Source: CAD feature listing. Evaluate the final solid. Frame: model axes, mm. Face numbers are marked on the shaded views. A direction names the side the tool comes from. Round coordinates to 2 decimals unless told otherwise and drop trailing zeros. Write each loop counter-clockwise with the first axis right and the second up, starting at its lowest first coordinate (ties: lowest second). Pieces come first, ordered by that corner, then holes. Notation, with made-up numbers: M 70,-31.5 L 83,-31.5 A21 ccw 83,-3.5 Z; hole C 21,-18.75 d5. An arc over 180 degrees is marked long. Answer in a Markdown table with one row per item.
from build123d import *

# Parameters (mm, degrees)
F0_W     = 30
F0_H     = 70
F1_DEPTH = 24
F2_W     = 60
F2_H     = 8.4
F3_DEPTH = 30.001
F5_DEPTH = 20
F6_W     = 20
F6_H     = 5
F7_DEPTH = 8
F9_DEPTH = 75
F10_R    = 5
F11_R    = 2.5
F12_R    = 2.5


with BuildPart() as f1:
    # F0 (on Top) → F1 (new body)
    with BuildSketch(Plane.XY):
        with Locations((15, -35)):
            Rectangle(F0_W, F0_H)
    extrude(amount=F1_DEPTH)

    # F2 (on face) → F3 (cut, through all)
    with BuildSketch(Plane(origin=(0, 0, 0), x_dir=(0, -1, 0), z_dir=(-1, 0, 0))):
        with Locations((40, 12.1)):
            Rectangle(F2_W, F2_H)
    extrude(amount=-F3_DEPTH, mode=Mode.SUBTRACT)

    # F4 (on Right) → F5 (join)
    with BuildSketch(Plane.YZ):
        Polygon((0, -145), (0, 0), (-12, 0), (-12, -92.6724137931), (-12, -125), (-12, -145), align=None)
        Polygon((-12, -125), (-12, -92.6724137931), (-55, 0), (-70, 0), align=None)
    extrude(amount=F5_DEPTH)

    # F6 (on face) → F7 (join)
    with BuildSketch(Plane(origin=(0, 0, 0), x_dir=(-1, 0, 0), z_dir=(0, 1, 0))):
        with Locations((-10, -142.5)):
            Rectangle(F6_W, F6_H)
    extrude(amount=F7_DEPTH)

    # F8 (on face) → F9 (cut)
    with BuildSketch(Plane.XY.offset(-140)):
        with BuildLine():
            ThreePointArc((0, -3.8196601125), (4.647668654, -0.9874146153), (10.0000000012, 0))
            Line((10.0000000012, 0), (0, 0))
            Line((0, 0), (0, -3.8196601125))
        make_face()
        with BuildLine():
            ThreePointArc((10.0000000012, 0), (15.6425875311, -1.1017552924), (20.4562749714, -4.2451725387))
            Line((20.4562749714, -4.2451725387), (20.4562749714, 0))
            Line((20.4562749714, 0), (20, 0))
            Line((20, 0), (10.0000000012, 0))
        make_face()
    extrude(amount=F9_DEPTH, mode=Mode.SUBTRACT)

    # F10
    f10_edges = [f1.edges().sort_by_distance(p)[0] for p in [
        (0, 8, -142.5),
        (20, 8, -142.5),
    ]]
    fillet(f10_edges, radius=F10_R)

    # F11
    f11_edges = [f1.edges().sort_by_distance(p)[0] for p in [
        (0, 0, -20.5),
        (20, 0, -32.5),
    ]]
    fillet(f11_edges, radius=F11_R)

    # F12
    f12_edges = [f1.edges().sort_by_distance(p)[0] for p in [
        (30, 0, 12),
    ]]
    fillet(f12_edges, radius=F12_R)


solid = f1.part
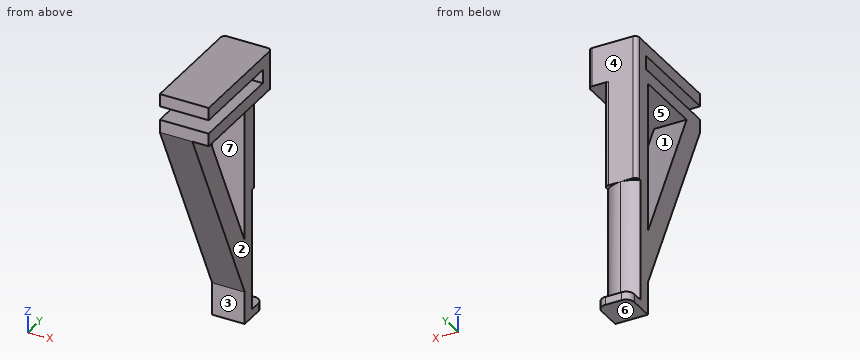
Q1. Pull-direction query (Y, two-part tool) for the marked faces 1, 2, 3 and 4; classes: pulls with the +Y half, pulls with the -Y half, needs draft (parallel to the pull), parting line crosses it, or undercut.
Solutions:
| item | result |
|---|---|
| face 1 | undercut |
| face 2 | needs draft |
| face 3 | pulls with the -Y half |
| face 4 | pulls with the +Y half |
Q2. Section C-C (y = -64). Return loops of the section in (x, z).
Solutions:
| item | result |
|---|---|
| outline | M 0,-12.93 L 20,-12.93 L 20,0 L 30,0 L 30,7.9 L 0,7.9 Z; M 0,16.3 L 30,16.3 L 30,24 L 0,24 Z |
Q3. Section A-A (y = -28.5). Return loops of the section in (x, z).
Solutions:
| item | result |
|---|---|
| outline | M 0,-89.44 L 20,-89.44 L 20,-57.11 L 0,-57.11 Z; M 0,0 L 30,0 L 30,7.9 L 0,7.9 Z; M 0,16.3 L 30,16.3 L 30,24 L 0,24 Z |
Q4. Section B-B (z = -54). Return loops of the section in (x, y).
Solutions:
| item | result |
|---|---|
| outline | M 0,-44.94 L 20,-44.94 L 20,-29.94 L 0,-29.94 Z; M 0,-12 L 20,-12 L 20,-2.5 A2.5 ccw 17.5,0 L 2.5,0 A2.5 ccw 0,-2.5 Z |
Q5. Material intervals for probe 1 along Z at (x, y) = (8.5, -41); probe 2 along Z at (x, y) = (11.5, -48.5); probe 3 along Z at (x, y) = (27, -15.5), sorted ascending.
Solutions:
| item | result |
|---|---|
| probe 1 | z = -62.5 to -30.17, 0 to 7.9, 16.3 to 24 |
| probe 2 | z = -46.34 to -14.01, 0 to 7.9, 16.3 to 24 |
| probe 3 | z = 0 to 7.9, 16.3 to 24 |
Q6. Contact query for flat-ended pins moving along their axis: pin 1 Ø6 at (x, z) = (5.5, -25.5) entering from -Y; pin 2 Ø1 at (y, z) = (-30, -66.5) entering from +X; pin 3 Ø3.5 at (x, y) = (8.5, 4) entering from +Z; pin 4 Ø9 at (x, z) = (20.5, 13.5) entering from -Y. Output: stop coordinate, or through.
Solutions:
| item | result |
|---|---|
| pin 1 | stops at y = -59.56 |
| pin 2 | stops at x = 20 |
| pin 3 | stops at z = -140 |
| pin 4 | stops at y = -70 |
Q7. Access query for the marked faces 5, 6 and 7. Directions: +Z, -Z, +X, -X, +Y, -Y. A direction counts if a zero-diameter tool reaches every point of the face in a straight line with its end or side. Return the directions, or none.
Solutions:
| item | result |
|---|---|
| face 5 | +X |
| face 6 | -Z, +X, -X, +Y, -Y |
| face 7 | +X, -X |
Q8. Section D-D (x = 7.5). Return loops of the section in (y, z), and give its area (3 significant figures).
Solutions:
| item | result |
|---|---|
| outline | M -70,0 L -12,-125 L -12,-145 L 8,-145 L 8,-140 L -0.21,-140 L -0.21,-65 L 0,-65 L 0,24 L -70,24 L -70,16.3 L -10,16.3 L -10,7.9 L -70,7.9 Z; hole M -55,0 L -12,-92.67 L -12,0 Z |
| area | 4,570 mm2 |
